Input: part model. Units: mm. Frame: model coordinates. Face numbers are marked on the shaded views. A direction names the side the tool comes from. Coordinates: 2 decimals unless noted, no trailing zeros. Loops run counter-clockwise (first coordinate to the right, second up) from the corner with the lowest first, then second, coordinate; pieces in that order, holes last. Notation, with made-up numbers: (19.25, -8) -> (39.25, -8) arc R5 ccw to (39.25, -4) -> close; hole circle Ø7 at (19, 23.25). An arc over 180 degrees is marked (long way). Answer as a JSON object with one key per item and string values.
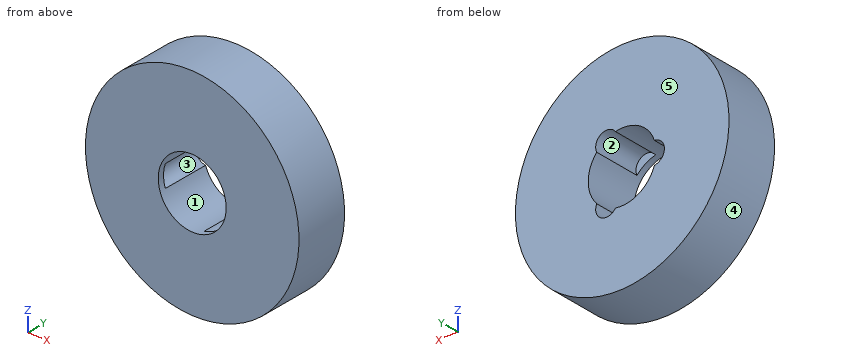
from build123d import *

# Parameters (mm, degrees)
SKETCH1_R           = 55
BOSS_EXTRUDE1_DEPTH = 27
SKETCH2_R           = 17.5
CUT_EXTRUDE1_DEPTH  = 83.33468285
SKETCH3_R           = 5.609144045
CUT_EXTRUDE2_DEPTH  = 23.860194
CIRPATTERN1_START   = 3.13980557
CIRPATTERN1_DEPTH   = 23.86019443


# Read off the part's stored shape, not the designer's step: CirPattern1
with BuildPart() as part:
    # Sketch1 → Boss-Extrude1 (new body)
    with BuildSketch(Plane(origin=(0, 0, 0), x_dir=(1, 0, 0), z_dir=(0, 1, 0))):
        with Locations(Location((0, 0, 0), (0, 0, 270))):
            Circle(SKETCH1_R)
    extrude(amount=BOSS_EXTRUDE1_DEPTH)

    # Sketch2 → Cut-Extrude1 (cut, through all)
    with BuildSketch(Plane(origin=(0, 0, 0), x_dir=(1, 0, 0), z_dir=(0, 1, 0))):
        with Locations(Location((0, 0, 0), (0, 0, 270))):
            Circle(SKETCH2_R)
    extrude(amount=CUT_EXTRUDE1_DEPTH, mode=Mode.SUBTRACT)

    # Sketch3 → Cut-Extrude2 (cut)
    with BuildSketch(Plane(origin=(0, 27, 0), x_dir=(1, 0, 0), z_dir=(0, 1, 0))):
        with Locations((-16.117619445, 0)):
            Circle(SKETCH3_R)
    extrude(amount=-CUT_EXTRUDE2_DEPTH, mode=Mode.SUBTRACT)

    # CirPattern1 outline → CirPattern1 (cut)
    with BuildSketch(Plane(origin=(0, 0, 0), x_dir=(1, 0, 0), z_dir=(0, 1, 0)).offset(CIRPATTERN1_START)):
        with BuildLine():
            ThreePointArc((3.450732443, 17.15641121), (8.75, 15.155444566), (13.132521724, 11.566627563))
            ThreePointArc((13.132521724, 11.566627563), (10.863381745, 18.815929125), (3.450732443, 17.15641121))
        make_face()
        with BuildLine():
            ThreePointArc((13.132521724, -11.566627563), (8.75, -15.155444566), (3.450732443, -17.15641121))
            ThreePointArc((3.450732443, -17.15641121), (10.863381745, -18.815929125), (13.132521724, -11.566627563))
        make_face()
    extrude(amount=CIRPATTERN1_DEPTH, mode=Mode.SUBTRACT)


solid = part.part
1. Pin query (flat end, axial travel): P1, Ø4, axis at x = -18.5, z = -0.5, coming from the +Y side; P2, Ø1, axis at x = 17, y = 15.5, coming from the +Z side; P3, Ø8, axis at x = -10.5, y = 14.5, coming from the +Z side. Return the tip coordinate at first contact, or that it passes through.
Reply:
{"P1": "stops at y = 3.14", "P2": "stops at z = 52.47", "P3": "stops at z = 54.61"}
2. Mould query, pull axis Z, two halves, no side actions, for the marked faces 3, 4 and 5. Classes: pulls with the +Z half, pulls with the -Z half, needs draft (parallel to the pull), parting line crosses it, or undercut.
Reply:
{"face 3": "undercut", "face 4": "parting line crosses it", "face 5": "needs draft"}
3. Section query D-D (z = -35). Return loops of the section in (x, y), plus the area to 3 significant figures.
Reply:
{"outline": "(-42.43, 0) -> (42.43, 0) -> (42.43, 27) -> (-42.43, 27) -> close", "area": "2,290 mm2"}
4. Section query B-B (x = 0). Return loops of the section in (y, z).
Reply:
{"outline": "(0, -55) -> (27, -55) -> (27, -17.5) -> (0, -17.5) -> close; (0, 17.5) -> (27, 17.5) -> (27, 55) -> (0, 55) -> close"}
5. Section query A-A (z = 0). Return loops of the section in (x, y).
Reply:
{"outline": "(-55, 0) -> (-17.5, 0) -> (-17.5, 3.14) -> (-21.73, 3.14) -> (-21.73, 27) -> (-55, 27) -> close; (17.5, 0) -> (55, 0) -> (55, 27) -> (17.5, 27) -> close"}
6. Access query for the marked faces 1 and 2. Directions: +Z, -Z, +X, -X, +Y, -Y. A direction counts if a zero-diameter tool reaches every point of the face in a straight line with its end or side. Return the directions, or none.
Reply:
{"face 1": "+Y, -Y", "face 2": "+Y"}
7. Section query C-C (y = 5). Return loops of the section in (x, z), plus the area to 3 significant figures.
Reply:
{"outline": "circle Ø110 at (0, 0); hole (-16.58, -5.59) arc R17.5 ccw to (3.45, -17.16) arc R5.61 ccw to (13.13, -11.57) arc R17.5 ccw to (13.13, 11.57) arc R5.61 ccw to (3.45, 17.16) arc R17.5 ccw to (-16.58, 5.59) arc R5.61 ccw to start", "area": "8,430 mm2"}
8. Line query: line 1 along X through (y, z) = (12.75, 0); line 2 along Z through (x, y) = (-11, 2.5); line 3 along Z through (x, y) = (-4, 25.5). Output: solid intervals per line, ascending.
Reply:
{"line 1": "x = -55 to -21.73, 17.5 to 55", "line 2": "z = -53.89 to -13.61, 13.61 to 53.89", "line 3": "z = -54.85 to -17.04, 17.04 to 54.85"}
